```python
from build123d import *

# Parameters (mm, degrees)
SKETCH1_W                      = 90
SKETCH1_H                      = 60
BOSS_EXTRUDE1_DEPTH            = 5
CBORE_FOR_M5_SHCS1_D           = 5.5
CBORE_FOR_M5_SHCS1_CBORE_D     = 10
CBORE_FOR_M5_SHCS1_CBORE_DEPTH = 5
LPATTERN1_COUNT                = 2
LPATTERN1_PITCH                = 60
LPATTERN1_COUNT_DIR2           = 2
LPATTERN1_PITCH_DIR2           = 40


with BuildPart() as part:
    # Sketch1 → Boss-Extrude1 (new body, symmetric)
    with BuildSketch(Plane.XY):
        Rectangle(SKETCH1_W, SKETCH1_H)
    extrude(amount=BOSS_EXTRUDE1_DEPTH, both=True)

    # CBORE for M5 SHCS1 (through all)
    with Locations(Plane.XY.offset(5)):
        with Locations((-25, 20)):
            cbore_for_m5_shcs1 = CounterBoreHole(CBORE_FOR_M5_SHCS1_D / 2, CBORE_FOR_M5_SHCS1_CBORE_D / 2, CBORE_FOR_M5_SHCS1_CBORE_DEPTH)

    # LPattern1: CBORE for M5 SHCS1 2 × 2
    with Locations(*[(i * LPATTERN1_PITCH, -j * LPATTERN1_PITCH_DIR2, 0) for i in range(LPATTERN1_COUNT) for j in range(LPATTERN1_COUNT_DIR2) if (i, j) != (0, 0)]):
        add(cbore_for_m5_shcs1, mode=Mode.SUBTRACT)


solid = part.part
```
Design review of the part built by this model. Coordinates are the model's own, in mm. A direction names the side the tool comes from. Coordinates: 2 decimals unless noted, no trailing zeros. Write each loop counter-clockwise with the first axis right and the second up, starting at its lowest first coordinate (ties: lowest second). Pieces come first, ordered by that corner, then holes. Notation, with made-up numbers: M 31,-5 L 86,-5 A33 cw 86,27 Z; hole C -31,-18.75 d1. An arc over 180 degrees is marked long. Answer as a JSON object with one key per item and string values.
Item 1: Add section C-C, the plane z = 3.75. Give the boundary of the cut face in (x, y).
Outcome:
{"outline": "M -45,-30 L 45,-30 L 45,30 L -45,30 Z; hole C -25,-20 d10; hole C -25,20 d10; hole C 35,-20 d10; hole C 35,20 d10"}
Item 2: Insertion check: pin 1 Ø6 at (x, y) = (-25, -20) entering from +Z. The pin has a flat end and moves straight along its axis. Give the tip position at first contact, or say it passes through.
Outcome:
{"pin 1": "z = 0"}
Item 3: Machinability: for faces 5 (the flat face through (-1, 0, -5)), 6 (the cylindrical face through (31, -23, 3)), which of the approach directions +Z, -Z, +X, -X, +Y, -Y give a long, thin tool a straight path to every point of the face, cutting with its end or side? Answer none if there is none.
Outcome:
{"face 5": "-Z, +X, -X, +Y, -Y", "face 6": "+Z"}
Item 4: Add section B-B, the plane y = -20. Give the boundary of the cut face in (x, z), and give its area (3 significant figures).
Outcome:
{"outline": "M -45,-5 L -27.75,-5 L -27.75,0 L -30,0 L -30,5 L -45,5 Z; M -22.25,-5 L 32.25,-5 L 32.25,0 L 30,0 L 30,5 L -20,5 L -20,0 L -22.25,0 Z; M 37.75,-5 L 45,-5 L 45,5 L 40,5 L 40,0 L 37.75,0 Z", "area": "745 mm²"}
Item 5: Draft analysis for pull direction X (two halves, no side actions). For faces 1 (the cylindrical face through (-29, 17, 3)), 2 (the cylindrical face through (-22.253, 20.121, -2.535)), 3 (the flat face through (-1, 0, 5)), 4 (the flat face through (45, 0, 0)), state which applies: pulls with the +X half, pulls with the -X half, needs draft (parallel to the pull), parting line crosses it, or undercut.
Outcome:
{"face 1": "undercut", "face 2": "undercut", "face 3": "needs draft", "face 4": "pulls with the +X half"}
Item 6: Wall thickness on probe 1 along Y at (x, z) = (-25, -1.5); probe 2 along Y at (x, z) = (35, 1.7); probe 3 along X at (y, z) = (19, -1.5): over which ranges is each line inside the solid? List them lowest first.
Outcome:
{"probe 1": "-30 to -22.75, -17.25 to 17.25, 22.75 to 30", "probe 2": "-30 to -25, -15 to 15, 25 to 30", "probe 3": "-45 to -27.56, -22.44 to 32.44, 37.56 to 45"}
Item 7: Add section A-A, the plane x = 35. Give the boundary of the cut face in (y, z).
Outcome:
{"outline": "M -30,-5 L -22.75,-5 L -22.75,0 L -25,0 L -25,5 L -30,5 Z; M -17.25,-5 L 17.25,-5 L 17.25,0 L 15,0 L 15,5 L -15,5 L -15,0 L -17.25,0 Z; M 22.75,-5 L 30,-5 L 30,5 L 25,5 L 25,0 L 22.75,0 Z"}
